Check sheet for the modelled part. Datum: model origin and axes. Units: mm. A direction names the side the tool comes from. Give positions to 0.01 mm unless a question says otherwise; leave off trailing zeros. Loops run counter-clockwise (first coordinate to the right, second up) from the corner with the lowest first, then second, coordinate; pieces in that order, holes last. Notation, with made-up numbers: M 84.25,29.25 L 122.25,29.25 A8 cw 122.25,38.25 Z; hole C 87.5,-13 d3. An arc over 180 degrees is marked long. Use one line per item in the form item = value.
from build123d import *

# Parameters (mm, degrees)
F0_W     = 23.1957846131
F0_H     = 3.81
F0_W_2   = 4.3642977253
F0_H_2   = 12.2541113061
F0_W_3   = 23.2399176616
F1_DEPTH = 2.54
F3_R     = 1.095
F3_R_2   = 1.1118429646
F5_DEPTH = 2.54
F6_W     = 40.64
F6_H     = 3.81
F7_DEPTH = 2.54
F8_R     = 1.095
F8_R_2   = 1.1118429646
F9_DEPTH = 2.54


with BuildPart() as f1:
    # F0 (on Front) → F1 (new body)
    with BuildSketch(Plane.XZ):
        with Locations((13.8021076934, 0)):
            Rectangle(F0_W, F0_H)
        with Locations((0.0220665243, 0)):
            Rectangle(F0_W_2, F0_H)
        with Locations((0.0220665243, 8.032055653)):
            Rectangle(F0_W_2, F0_H_2)
        with Locations((-13.7800411692, 0)):
            Rectangle(F0_W_3, F0_H)
    extrude(amount=F1_DEPTH)


with BuildPart() as f1_1:
    # F2: moved
    add(f1.part.moved(Location((0, -20.32, 0))))


with BuildPart() as f4_1:
    # F4: instance of F1
    add(f1_1.part.mirror(Plane.XZ))


with BuildPart() as f1_2:
    add(f1_1.part)

    # F3 (on face) → F5 (cut, through all)
    with BuildSketch(Plane.XZ.offset(22.86)):
        with Locations((7.615, 0)):
            Circle(F3_R)
        with Locations((17.785, 0)):
            Circle(F3_R)
        with Locations((0, 10)):
            Circle(F3_R_2)
    extrude(amount=-F5_DEPTH, mode=Mode.SUBTRACT)

    add(f4_1.part)  # F7 merges F4_1
    # F6 (on face) → F7 (join)
    with BuildSketch(Plane.YZ.offset(25.4)):
        Rectangle(F6_W, F6_H)
    extrude(amount=-F7_DEPTH)

    # F8 (on face) → F9 (cut, through all)
    with BuildSketch(Plane(origin=(0, 22.86, 0), x_dir=(-1, 0, 0), z_dir=(0, 1, 0))):
        with Locations((7.615, 0)):
            Circle(F8_R)
        with Locations((17.785, 0)):
            Circle(F8_R)
        with Locations((0, 10)):
            Circle(F8_R_2)
    extrude(amount=-F9_DEPTH, mode=Mode.SUBTRACT)


solid = f1_2.part
1) Scan lines: line 1 (Z direction, x = 0, y = 21.5) (3 decimals); line 2 (Y direction, x = -7, z = -1); line 3 (Z direction, x = 18, y = 20.5) (3 decimals). Record each from-to range of solid material in increasing order.
Evaluation:
line_1 = -1.905 to 8.888, 11.112 to 14.159
line_2 = -22.86 to -20.32, 20.32 to 22.86
line_3 = -1.905 to 1.905
2) Section check B-B (z = 10). Record the cut outline in (x, y), then the cut area to 3 significant figures.
Evaluation:
outline = M -2.16,-22.86 L -1.11,-22.86 L -1.11,-20.32 L -2.16,-20.32 Z; M -2.16,20.32 L -1.11,20.32 L -1.11,22.86 L -2.16,22.86 Z; M 1.11,-22.86 L 2.2,-22.86 L 2.2,-20.32 L 1.11,-20.32 Z; M 1.11,20.32 L 2.2,20.32 L 2.2,22.86 L 1.11,22.86 Z
area = 10.9 mm^2
3) Release check for a two-part mould opening along Z. For faces 4 (the face through (0, 22, 14.159)), 5 (the face through (-2.16, 22, 8)), 6 (the face through (8.66, -21.61, 0.33)) record: pulls with the +Z half, pulls with the -Z half, needs draft (parallel to the pull), parting line crosses it, or undercut.
Evaluation:
face_4 = pulls with the +Z half
face_5 = needs draft
face_6 = undercut
4) Set-up check for faces 1 (the face through (-14, 22, 1.905)), 2 (the face through (-8.66, 21.61, 0.33)), 3 (the face through (22.86, 0, 0)): record each of +Z, -Z, +X, -X, +Y, -Y from which the full face is reachable in a straight line by a thin tool's end or side.
Evaluation:
face_1 = +Z, -X, +Y, -Y
face_2 = +Y
face_3 = +Z, -Z, -X
5) Section check D-D (x = 0). Record the cut outline in (y, z) (3 decimals).
Evaluation:
outline = M -22.86,-1.905 L -20.32,-1.905 L -20.32,8.888 L -22.86,8.888 Z; M -22.86,11.112 L -20.32,11.112 L -20.32,14.159 L -22.86,14.159 Z; M 20.32,-1.905 L 22.86,-1.905 L 22.86,8.888 L 20.32,8.888 Z; M 20.32,11.112 L 22.86,11.112 L 22.86,14.159 L 20.32,14.159 Z
6) Depth check by flat-ended pin: pin 1 Ø2 at (x, y) = (-18.5, -22) entering from +Z (3 decimals); pin 2 Ø0.8 at (y, z) = (22, 6) entering from +X; pin 3 Ø7 at (x, y) = (18, 10) entering from +Z; pin 4 Ø3 at (y, z) = (21.5, 10.5) entering from -X. Enter the tip coordinate at first touch or a pass-through.
Evaluation:
pin_1 = 1.905
pin_2 = 2.2
pin_3 = through
pin_4 = -2.16
7) Section check C-C (z = 5.5). Record the cut outline in (x, y), then the cut area to 3 significant figures.
Evaluation:
outline = M -2.16,-22.86 L 2.2,-22.86 L 2.2,-20.32 L -2.16,-20.32 Z; M -2.16,20.32 L 2.2,20.32 L 2.2,22.86 L -2.16,22.86 Z
area = 22.2 mm^2
8) Section check A-A (x = 11). Record the cut outline in (y, z) (3 decimals).
Evaluation:
outline = M -22.86,-1.905 L -20.32,-1.905 L -20.32,1.905 L -22.86,1.905 Z; M 20.32,-1.905 L 22.86,-1.905 L 22.86,1.905 L 20.32,1.905 Z
